from build123d import *

# Parameters (mm, degrees)
SKETCH_1_W                       = 564
SKETCH_1_H                       = 50
SM_BASE_FLANGE_1_DEPTH           = 2
SM_EDGE_FLANGE_1_STRIP_W         = 12
SM_EDGE_FLANGE_1_STRIP_H         = 2
SM_EDGE_FLANGE_1_STRIP_CUT_DEPTH = 50
SM_EDGE_FLANGE_1_DEPTH           = 50
SM_EDGE_FLANGE_2_STRIP_W         = 12
SM_EDGE_FLANGE_2_STRIP_H         = 2
SM_EDGE_FLANGE_2_STRIP_CUT_DEPTH = 50
SM_EDGE_FLANGE_2_DEPTH           = 50


# Sheet-metal steps are written as plain solids
with BuildPart() as part:
    # Sketch 1 → Базовая кромка1 (new body)
    with BuildSketch(Plane.XY):
        with Locations((282, 25)):
            Rectangle(SKETCH_1_W, SKETCH_1_H)
    extrude(amount=SM_BASE_FLANGE_1_DEPTH)

    # Ребро-кромка1 strip (across the edge) → Ребро-кромка1 strip cut (cut)
    with BuildSketch(Plane(origin=(0, 50, 2), x_dir=(1, 0, 0), z_dir=(0, -1, 0))):
        with Locations((-2, -1)):
            Rectangle(SM_EDGE_FLANGE_1_STRIP_W, SM_EDGE_FLANGE_1_STRIP_H)
    extrude(amount=SM_EDGE_FLANGE_1_STRIP_CUT_DEPTH, mode=Mode.SUBTRACT)

    # Ребро-кромка1 section (across the edge) → Ребро-кромка1 (add)
    with BuildSketch(Plane(origin=(0, 50, 2), x_dir=(1, 0, 0), z_dir=(0, -1, 0))):
        with BuildLine():
            Line((0, 2), (0, 48))
            Line((0, 48), (2, 48))
            Line((2, 48), (2, 2))
            ThreePointArc((2, 2), (2.585786438, 0.585786438), (4, 0))
            Line((4, 0), (4, -2))
            ThreePointArc((4, -2), (1.171572875, -0.828427125), (0, 2))
        make_face()
    extrude(amount=SM_EDGE_FLANGE_1_DEPTH)

    # Ребро-кромка2 strip (across the edge) → Ребро-кромка2 strip cut (cut)
    with BuildSketch(Plane(origin=(564, 0, 2), x_dir=(-1, 0, 0), z_dir=(0, 1, 0))):
        with Locations((-2, -1)):
            Rectangle(SM_EDGE_FLANGE_2_STRIP_W, SM_EDGE_FLANGE_2_STRIP_H)
    extrude(amount=SM_EDGE_FLANGE_2_STRIP_CUT_DEPTH, mode=Mode.SUBTRACT)

    # Ребро-кромка2 section (across the edge) → Ребро-кромка2 (add)
    with BuildSketch(Plane(origin=(564, 0, 2), x_dir=(-1, 0, 0), z_dir=(0, 1, 0))):
        with BuildLine():
            Line((0, 2), (0, 48))
            Line((0, 48), (2, 48))
            Line((2, 48), (2, 2))
            ThreePointArc((2, 2), (2.585786438, 0.585786438), (4, 0))
            Line((4, 0), (4, -2))
            ThreePointArc((4, -2), (1.171572875, -0.828427125), (0, 2))
        make_face()
    extrude(amount=SM_EDGE_FLANGE_2_DEPTH)


solid = part.part
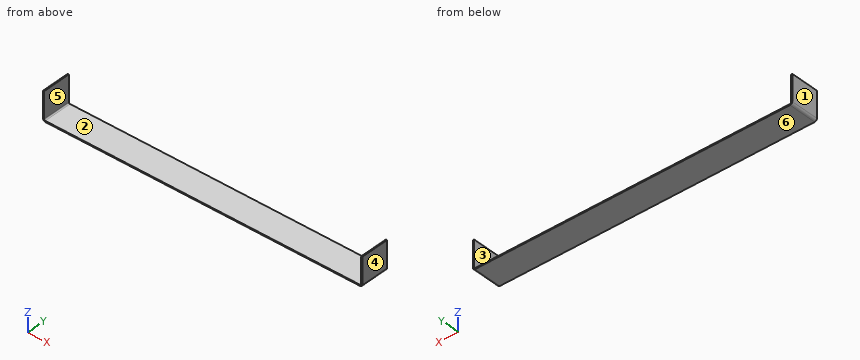
Can you work these out from the model? Positions are in its coordinate system, mm. Face numbers are marked on the shaded views. A direction names the side the tool comes from. Round coordinates to 2 decimals unless told otherwise and drop trailing zeros. Write each loop counter-clockwise with the first axis right and the second up, starting at its lowest first coordinate (ties: lowest second). Pieces come first, ordered by that corner, then holes. Notation, with made-up numbers: (-27, 66.25) -> (-1, 66.25) arc R31 cw to (-1, 90.25) -> close; hole circle Ø9 at (83.25, 19.5). An arc over 180 degrees is marked (long way). Use one line per item in the form item = value. Start each with the question number.
Q1. We'd pull the mould along X, two halves only. Please class the marked faces 3, 4, 5 and 6: +X half, -X half, draft (parallel to the pull), parting line (faces both ways), or undercut.
Q2. Which directions (+Z, -Z, +X, -X, +Y, -Y) give clear straight access to the entire face, cutting with the end or side of a thin tool? Please do the marked faces 1 and 2.
Q3. Imagine slicing it at C-C (x = 520). Please give me the cut outline in (y, z).
Q4. Imagine slicing it at B-B (y = 38). Please give me the cut outline in (x, z), then the cut area to 3 significant figures.
Q5. Imagine slicing it at A-A (z = 37). Please give me the cut outline in (x, y).
Q6. If I drill on probe 1 along X at (y, z) = (15, 48); probe 2 along Z at (x, y) = (32.5, 17), over which ranges is the centre line in solid material (lowest first)? Write a range as [from, to].
Q7. I'm going to push a flat-ended pin straight in: P1, Ø2, axis at x = 449.5, y = 42, coming from the +Z side. Where does the tip first touch, or does it pass through?
Worked out:
q1.face_3 = undercut
q1.face_4 = +X half
q1.face_5 = undercut
q1.face_6 = draft
q2.face_1 = +Z, -Z, -X, +Y, -Y
q2.face_2 = +Z, +Y, -Y
q3.outline = (0, 0) -> (50, 0) -> (50, 2) -> (0, 2) -> close
q4.outline = (0, 4) arc R4 ccw to (4, 0) -> (560, 0) arc R4 ccw to (564, 4) -> (564, 50) -> (562, 50) -> (562, 4) arc R2 cw to (560, 2) -> (4, 2) arc R2 cw to (2, 4) -> (2, 50) -> (0, 50) -> close
q4.area = 1,310 mm^2
q5.outline = (0, 0) -> (2, 0) -> (2, 50) -> (0, 50) -> close; (562, 0) -> (564, 0) -> (564, 50) -> (562, 50) -> close
q6.probe_1 = [0, 2], [562, 564]
q6.probe_2 = [0, 2]
q7.P1 = 2
